Autodesk Inventor part; units mm, degrees
ref_plane "YZ Plane" through (0, 0, 0) normal (1, 0, 0) x (0, 1, 0)
ref_plane "XZ Plane" through (0, 0, 0) normal (0, 1, 0) x (-1, 0, 0)
ref_plane "XY Plane" through (0, 0, 0) normal (0, 0, 1) x (1, 0, 0)
sketch "Sketch1" plane through (0, 0, 0) normal (0, 0, 1) x (1, 0, 0)
  line L0 (0, 0) -> (5.8, 0) construction
  line L1 (5.8, 0) -> (5.8, 4.3) construction
  line L2 (5.8, 4.3) -> (0, 4.3) construction
  line L3 (0, 4.3) -> (0, 0) construction
  line L4 (5.8, 4.3) -> (-5.5, 4.3)
  line L5 (-5.5, 4.3) -> (-5.5, -4.3)
  line L6 (-5.5, -4.3) -> (5.8, -4.3)
  line L7 (5.8, -4.3) -> (5.8, 4.3)
  dimension "d0" = 5.8
  dimension "d1" = 4.3
  dimension "d2" = 11.3
  dimension "d3" = 8.6
extrude "Extrusion1" add sketch "Sketch1" along normal blind 4
sketch "Sketch2" plane through (0, 0, 0) normal (0, 0, -1) x (-1, 0, 0)
  line L0 (-5.8, 4.3) -> (5.5, 4.3)
  line L1 (5.5, -4.3) -> (4, -4.3) construction
  line L2 (4, -4.3) -> (4, 4.3) construction
  line L3 (4, 4.3) -> (5.5, 4.3) construction
  line L4 (5.5, 4.3) -> (5.5, -4.3) construction
  line L5 (4, -4.3) -> (-5.8, -4.3)
  line L6 (-5.8, -4.3) -> (-5.8, 4.3)
  line L7 (-5.8, 4.3) -> (4, 4.3)
  line L8 (4, 4.3) -> (4, -4.3)
  point P0 (0, 0)
  dimension "d6" = 1.5
extrude "Extrusion2" cut sketch "Sketch2" against normal blind 1.45
sketch "Sketch3" plane through (0, 0, 1.45) normal (0, 0, -1) x (-1, 0, 0)
  line L0 (4, -4.3) -> (4, 4.3)
  line L1 (-5.8, -4.3) -> (-5.4, -4.3) construction
  line L2 (-5.4, -4.3) -> (-5.4, -3.9) construction
  line L3 (-5.4, -3.9) -> (-5.8, -3.9) construction
  line L4 (-5.8, -3.9) -> (-5.8, -4.3) construction
  line L5 (-5.8, 4.3) -> (-5.4, 4.3) construction
  line L6 (-5.4, 4.3) -> (-5.4, 3.9) construction
  line L7 (-5.4, 3.9) -> (-5.8, 3.9) construction
  line L8 (-5.8, 3.9) -> (-5.8, 4.3) construction
  line L9 (-5.4, -3.9) -> (4, -3.9)
  line L10 (4, -3.9) -> (4, 3.9)
  line L11 (4, 3.9) -> (-5.4, 3.9)
  line L12 (-5.4, 3.9) -> (-5.4, -3.9)
  point P0 (0, 0)
  dimension "d9" = 0.4
  dimension "d10" = 0.4
  dimension "d11" = 0.4
  dimension "d12" = 0.4
extrude "Extrusion3" cut sketch "Sketch3" against normal blind 0.8
properties part number "lid_f"
Build history of the part. All positions in model axes, mm. A direction names the side the tool comes from. Round coordinates to 2 decimals unless told otherwise and drop trailing zeros. Loops run counter-clockwise (first coordinate to the right, second up) from the corner with the lowest first, then second, coordinate; pieces in that order, holes last.
Item 1: Drill centre lines: line 1 along Y through (x, z) = (5, 2.15); line 2 along X through (y, z) = (-3.25, 1.85); line 3 along Z through (x, y) = (3, -2.5). Where is each one in solid material? Low to high.
Item 2: Saw through at D-D (z = 0.85). List the corners of the cut face in (x, y).
Item 3: Two-plate mould, pull along Y, no slides. Class faces 1 (the face through (0, 4.3, 2)), 2 (the face through (-4, 0, 1)), 3 (the face through (0, -4.3, 2)): released by +Y, released by -Y, zero draft, split by the parting line, or undercut.
Item 4: Saw through at A-A (x = -1.25). List the corners of the cut face in (y, z).
Item 5: Which spindle directions (+Z, -Z, +X, -X, +Y, -Y) get a long thin tool onto all of the face, cutting with end or side? Do faces 4 (the face through (0, 0, 4)), 5 (the face through (1, 0, 2.25)), 6 (the face through (5.6, 0, 1.45)). Say none if no direction does.
Item 6: Pin check, flat tip, straight feed: P1, Ø4.5, axis at x = 0.5, y = -1, coming from the -Z side. Stop position of the tip, or through.
Item 7: Saw through at C-C (z = 1.95). List the corners of the cut face in (x, y).
Item 8: Saw through at B-B (y = 2). List the corners of the cut face in (x, z).
Worked answers:
1. line 1: y = -4.3 to -3.9, 3.9 to 4.3
1. line 2: x = -5.5 to -4, 5.4 to 5.8
1. line 3: z = 2.25 to 4
2. outline: (-5.5, -4.3) - (-4, -4.3) - (-4, 4.3) - (-5.5, 4.3) - close
3. face 1: released by +Y
3. face 2: undercut
3. face 3: released by -Y
4. outline: (-4.3, 1.45) - (-3.9, 1.45) - (-3.9, 2.25) - (3.9, 2.25) - (3.9, 1.45) - (4.3, 1.45) - (4.3, 4) - (-4.3, 4) - close
5. face 4: +Z, +X, -X, +Y, -Y
5. face 5: -Z
5. face 6: -Z, +X, +Y, -Y
6. P1: stops at z = 2.25
7. outline: (-5.5, -4.3) - (5.8, -4.3) - (5.8, 4.3) - (-5.5, 4.3) - close; hole (-4, -3.9) - (5.4, -3.9) - (5.4, 3.9) - (-4, 3.9) - close
8. outline: (-5.5, 0) - (-4, 0) - (-4, 2.25) - (5.4, 2.25) - (5.4, 1.45) - (5.8, 1.45) - (5.8, 4) - (-5.5, 4) - close
